Could you check a few things on this model? Use its own coordinates, in mm. A direction names the side the tool comes from. Give positions to 0.01 mm unless a question says otherwise; leave off trailing zeros. Write each loop counter-clockwise with the first axis right and the second up, starting at its lowest first coordinate (ties: lowest second). Pieces come first, ordered by that corner, then holes. Notation, with made-up numbers: (81.25, -36.5) - (109.25, -36.5) arc R22 ccw to (109.25, -30.5) - close; hole circle Ø9 at (-31, -2.75). An arc over 180 degrees is marked (long way). Use one line per item in the form item = value.
```python
from build123d import *

# Parameters (mm, degrees)
SKETCH_1_R                   = 14
EXTRUDE_1_DEPTH              = 8
SKETCH_2_R                   = 11
EXTRUDE_2_DEPTH              = 3.5
HOLE_WIZARD_M8_1_D           = 9
HOLE_WIZARD_M8_1_CBORE_D     = 15
HOLE_WIZARD_M8_1_CBORE_DEPTH = 8.6
CHAMFER_1_SIZE               = 0.5


with BuildPart() as part:
    # 草圖1 → 填料-伸長1 (new body)
    with BuildSketch(Plane(origin=(0, 0, 0), x_dir=(1, 0, 0), z_dir=(0, 1, 0))):
        with Locations(Location((0, 0, 0), (0, 0, 270))):
            Circle(SKETCH_1_R)
    extrude(amount=EXTRUDE_1_DEPTH)

    # 草圖2 → 填料-伸長2 (add)
    with BuildSketch(Plane(origin=(0, 8, 0), x_dir=(1, 0, 0), z_dir=(0, 1, 0))):
        with Locations(Location((0, 0, 0), (0, 0, 270))):
            Circle(SKETCH_2_R)
    extrude(amount=EXTRUDE_2_DEPTH)

    # M8 六角承窩頭蓋螺釘的柱孔1 (through all)
    with Locations(Plane(origin=(0, 0, 0), x_dir=(-1, 0, 0), z_dir=(0, -1, 0))):
        with Locations((0, 0)):
            CounterBoreHole(HOLE_WIZARD_M8_1_D / 2, HOLE_WIZARD_M8_1_CBORE_D / 2, HOLE_WIZARD_M8_1_CBORE_DEPTH)

    # 導角1
    chamfer_1_edges = [part.edges().sort_by_distance(p)[0] for p in [
        (0, 11.5, -11),
    ]]
    chamfer(chamfer_1_edges, length=CHAMFER_1_SIZE)


solid = part.part
```
1. For pin 1 (5 mm diameter, centred on y = 4.5, z = 10, fed in from -X); pin 2 (12 mm diameter, centred on x = 2, z = -0.5, fed in from -Y); pin 3 (5 mm diameter, centred on y = 7, z = 7, fed in from +X); pin 4 (5 mm diameter, centred on y = 9, z = -4, fed in from -X), each with a flat end and sliding along its axis, tell me the tip position at first contact or that it passes through.
Response values:
pin_1 = -11.82
pin_2 = 0
pin_3 = 13.26
pin_4 = -13.9
2. If we mould it in two halves opening along X, with no side actions, what happens to faces 1 (the face through (0, 8.6, 5)), 2 (the face through (-6, 0, 6)), 3 (the face through (-13.67, 3.94, -3.03))? For each: pulls with the +X half, pulls with the -X half, needs draft (parallel to the pull), parting line crosses it, or undercut.
Response values:
face_1 = undercut
face_2 = needs draft
face_3 = parting line crosses it
3. Imagine slicing it at B-B, the plane z = 0. List the corners of the cut face in (x, y) for me, and give its area (3 significant figures).
Response values:
outline = (-14, 0) - (-7.5, 0) - (-7.5, 8.6) - (-4.5, 8.6) - (-4.5, 11.5) - (-10.5, 11.5) - (-11, 11) - (-11, 8) - (-14, 8) - close; (4.5, 8.6) - (7.5, 8.6) - (7.5, 0) - (14, 0) - (14, 8) - (11, 8) - (11, 11) - (10.5, 11.5) - (4.5, 11.5) - close
area = 146 mm²
4. Imagine slicing it at C-C, the plane y = 5.25. List the corners of the cut face in (x, z) for me.
Response values:
outline = circle Ø28 at (0, 0); hole circle Ø15 at (0, 0)
5. Which directions (+Z, -Z, +X, -X, +Y, -Y) give clear straight access to the entire face, cutting with the end or side of a thin tool? Please do faces 4 (the face through (7.493, 4.24, -0.33)), 5 (the face through (-0.59, 10.07, -4.46)), 6 (the face through (-10.74, 9.48, -2.38)).
Response values:
face_4 = -Y
face_5 = +Y, -Y
face_6 = +Y
6. Imagine slicing it at A-A, the plane x = 0. List the corners of the cut face in (y, z) for me.
Response values:
outline = (0, -14) - (8, -14) - (8, -11) - (11, -11) - (11.5, -10.5) - (11.5, -4.5) - (8.6, -4.5) - (8.6, -7.5) - (0, -7.5) - close; (0, 7.5) - (8.6, 7.5) - (8.6, 4.5) - (11.5, 4.5) - (11.5, 10.5) - (11, 11) - (8, 11) - (8, 14) - (0, 14) - close
7. If I drill on line 1 (Y direction, x = 0.5, z = 6); line 2 (Z direction, x = 2.5, y = 6.75); line 3 (Y direction, x = -8.75, z = 9.5), over which ranges is the centre line in solid material (lowest first)? Write a range as from..to.
Response values:
line_1 = 8.6..11.5
line_2 = -13.77..-7.07, 7.07..13.77
line_3 = 0..8
